```python
from build123d import *

# Parameters (mm, degrees)
BOSS_EXTRUDE1_DEPTH             = 6.35
FILLET1_R                       = 6.35
TAP_DRILL_FOR_1_4_20_TAP1_D     = 5.1054
TAP_DRILL_FOR_1_4_20_TAP1_DEPTH = 12.7
TAP_DRILL_FOR_1_4_20_TAP1_TIP   = 1.533816902
TAP_DRILL_FOR_1_4_20_TAP2_D     = 5.1054
TAP_DRILL_FOR_1_4_20_TAP2_DEPTH = 12.7
TAP_DRILL_FOR_1_4_20_TAP2_TIP   = 1.533816902


with BuildPart() as part:
    # Sketch1 → Boss-Extrude1 (new, symmetric)
    with BuildSketch(Plane.XY):
        Polygon((0, 12.7), (0, -12.7), (-27.578975516, -12.7), (-57.8104, -42.931424484), (-57.8104, -172.72), (-83.2104, -172.72), (-83.2104, -32.4104), (-38.1, 12.7), align=None)
    extrude(amount=BOSS_EXTRUDE1_DEPTH, both=True)

    # Fillet1
    fillet1_edges = [part.edges().sort_by_distance(p)[0] for p in [
        (-27.578975516, -12.7, 0),
        (-57.8104, -42.931424484, 0),
        (-83.2104, -32.4104, 0),
        (-38.1, 12.7, 0),
    ]]
    fillet(fillet1_edges, radius=FILLET1_R)

    # Tap Drill for 1/4-20 Tap1
    with Locations(Plane(origin=(0, 0, 0), x_dir=(0, 0, -1), z_dir=(1, 0, 0))):
        with Locations((0, 0)):
            Hole(TAP_DRILL_FOR_1_4_20_TAP1_D / 2, depth=TAP_DRILL_FOR_1_4_20_TAP1_DEPTH)
            with Locations((0, 0, -(TAP_DRILL_FOR_1_4_20_TAP1_DEPTH + TAP_DRILL_FOR_1_4_20_TAP1_TIP / 2))):  # 118° drill point
                Cone(0, TAP_DRILL_FOR_1_4_20_TAP1_D / 2, TAP_DRILL_FOR_1_4_20_TAP1_TIP, mode=Mode.SUBTRACT)

    # Tap Drill for 1/4-20 Tap2
    with Locations(Plane(origin=(0, -172.72, 0), x_dir=(-1, 0, 0), z_dir=(0, -1, 0))):
        with Locations((70.5104, 0)):
            Hole(TAP_DRILL_FOR_1_4_20_TAP2_D / 2, depth=TAP_DRILL_FOR_1_4_20_TAP2_DEPTH)
            with Locations((0, 0, -(TAP_DRILL_FOR_1_4_20_TAP2_DEPTH + TAP_DRILL_FOR_1_4_20_TAP2_TIP / 2))):  # 118° drill point
                Cone(0, TAP_DRILL_FOR_1_4_20_TAP2_D / 2, TAP_DRILL_FOR_1_4_20_TAP2_TIP, mode=Mode.SUBTRACT)


solid = part.part
```
Here's how the part is built. I have some questions about the finished solid (model axes, mm). A direction names the side the tool comes from. Coordinates: 2 decimals unless noted, no trailing zeros. Order: outer loops, then holes, each group sorted by start corner. A loop starts at its lowest first (then second) coordinate and runs counter-clockwise, first axis right, second up.
Item 1: I need wall thicknesses on probe 1 along Y at (x, z) = (-2.25, 0); probe 2 along X at (y, z) = (-80, -4); probe 3 along Y at (x, z) = (-24.5, 3.75). Which ranges of each line are inside material? Lowest first, please.
Response values:
probe 1: y = -12.7 to -2.55, 2.55 to 12.7
probe 2: x = -83.21 to -57.81
probe 3: y = -12.7 to 12.7
Item 2: Thinking about a two-plate mould opening in Z: for faces 6 (the face through (-70.16, -158.75, 0.27)), 7 (the face through (-82.714, -32.578, 0.089)), 8 (the face through (-60, -73, -6.35)), which applies, pulls with the +Z half, pulls with the -Z half, needs draft (parallel to the pull), parting line crosses it, or undercut?
Response values:
face 6: undercut
face 7: needs draft
face 8: pulls with the -Z half
Item 3: If we section it at A-A, the plane x = -6.5: List the corners of the cut face in (y, z) for me.
Response values:
outline: (-12.7, -6.35) - (12.7, -6.35) - (12.7, 6.35) - (-12.7, 6.35) - close; hole circle Ø5.11 at (0, 0)
Item 4: I'm going to push flat-ended pins straight in: pin 1 Ø3 at (x, z) = (-70.51, 0) entering from -Y; pin 2 Ø6 at (y, z) = (0, 0) entering from +X; pin 3 Ø4 at (y, z) = (-11, -1.5) entering from -X; pin 4 Ø4 at (y, z) = (-136, -2) entering from +X. Where does each tip first touch, or does it pass through?
Response values:
pin 1: stops at y = -159.39
pin 2: stops at x = 0
pin 3: stops at x = -63.8
pin 4: stops at x = -57.81
Item 5: Which directions (+Z, -Z, +X, -X, +Y, -Y) give clear straight access to the entire face, cutting with the end or side of a thin tool? Please do faces 1 (the face through (-12, -12.7, 0)), 2 (the face through (-73.06, -166.28, -0.11)), 3 (the face through (-6.439, 0.767, 2.435)), 4 (the face through (-60.9, -10.1, 0.1)), 5 (the face through (-83.21, -105, 0)).
Response values:
face 1: +Z, -Z, +X, -Y
face 2: -Y
face 3: +X
face 4: +Z, -Z, -X, +Y
face 5: +Z, -Z, -X, +Y, -Y
Item 6: If we section it at C-C, the plane y = -103: List the corners of the cut face in (x, z) for me, then the cut area to 3 significant figures.
Response values:
outline: (-83.21, -6.35) - (-57.81, -6.35) - (-57.81, 6.35) - (-83.21, 6.35) - close
area: 323 mm2
Item 7: If we section it at B-B, the plane x = -19: List the corners of the cut face in (y, z) for me.
Response values:
outline: (-12.7, -6.35) - (12.7, -6.35) - (12.7, 6.35) - (-12.7, 6.35) - close
